Geometry check sheet. Reference: the model listing, model coordinates, mm. A direction names the side the tool comes from. Coordinates: 2 decimals unless noted, no trailing zeros. Write each loop counter-clockwise with the first axis right and the second up, starting at its lowest first coordinate (ties: lowest second). Pieces come first, ordered by that corner, then holes. Notation, with made-up numbers: (12.5, 42.25) -> (69.5, 42.25) arc R26 cw to (69.5, 70.25) -> close; hole circle Ø9 at (-11, 70). An arc over 180 degrees is marked (long way). Answer in a Markdown table with one row per item. Add a question column.
Q1. Gauge pin test, flat end, axial feed: P1, Ø2, axis at x = 0, y = -22.225, coming from the -Z side. Record the tip position at first contact, or that the pin passes through.
Q2. Section check C-C, the plane z = 3. Count the separate pieces of the cut face and the enclosed holes in it, and give its area (3 significant figures).
Q3. Release check for a two-part mould opening along X. For faces 1 (the face through (-20.3, -20.11, 2.57)), 2 (the face through (12, -12, 5.207)), 3 (the face through (20.11, -20.3, 2.57)), 4 (the face through (16.71, 16.63, 2.57)) record: pulls with the +X half, pulls with the -X half, needs draft (parallel to the pull), parting line crosses it, or undercut.
Q4. Section check D-D, the plane y = 24.5. Record the boundary of the cut face in (x, z), and give its area (3 significant figures).
Q5. Tool access check on faces 5 (the face through (20.9, 7.283, 2.64)), 6 (the face through (12, -12, 0)). Record the directions out of +Z, -Z, +X, -X, +Y, -Y that give a thin tool (end or side, any length) a straight path to the whole face; none if there is none.
Q6. Thickness scan on line 1 (Y direction, x = 0, z = 3.1) (3 decimals); line 2 (Y direction, x = 21, z = 0.35); line 3 (Y direction, x = -7.5, z = 0.8). Record the ranges inside material, lowest first.
Q7. Section check A-A, the plane x = 0. Record the boundary of the cut face in (y, z) (3 decimals), and give its area (3 significant figures).
```python
from build123d import *

# Parameters (mm, degrees)
SKETCH4_R             = 28.575
BOSS_EXTRUDE2_DEPTH   = 5.207
SKETCH5_R             = 15.875
CUT_EXTRUDE5_DEPTH    = 6.207
CUT_EXTRUDE11_DEPTH   = 6.207
F_6_32_TAPPED_HOLE1_D = 2.7051


with BuildPart() as part:
    # Sketch4 → Boss-Extrude2 (new body)
    with BuildSketch(Plane.XY):
        Circle(SKETCH4_R)
    extrude(amount=BOSS_EXTRUDE2_DEPTH)

    # Sketch5 → Cut-Extrude5 (cut, through all)
    with BuildSketch(Plane.XY.offset(5.207)):
        Circle(SKETCH5_R)
    extrude(amount=-CUT_EXTRUDE5_DEPTH, mode=Mode.SUBTRACT)

    # Sketch8 → Cut-Extrude11 (cut, through all)
    with BuildSketch(Plane.XY.offset(5.207)):
        Polygon((32.367148217, 14.781549861), (13.593916116, 7.005422516), (14.565932035, 4.658768503), (33.339164135, 12.434895849), align=None)
        Polygon((12.351510066, 26.500513186), (10.004856053, 27.472529104), (9.518848094, 26.299202097), (11.865502107, 25.327186179), align=None)
        Polygon((-10.004856053, 27.472529104), (-12.351510066, 26.500513186), (-11.865502107, 25.327186179), (-9.518848094, 26.299202097), align=None)
        Polygon((-26.500513186, 12.351510066), (-27.472529104, 10.004856053), (-26.299202097, 9.518848094), (-25.327186179, 11.865502107), align=None)
        Polygon((-27.472529104, -10.004856053), (-26.500513186, -12.351510066), (-25.327186179, -11.865502107), (-26.299202097, -9.518848094), align=None)
        Polygon((-12.351510066, -26.500513186), (-10.004856053, -27.472529104), (-9.518848094, -26.299202097), (-11.865502107, -25.327186179), align=None)
        Polygon((10.004856053, -27.472529104), (12.351510066, -26.500513186), (11.865502107, -25.327186179), (9.518848094, -26.299202097), align=None)
        Polygon((26.500513186, -12.351510066), (27.472529104, -10.004856053), (26.299202097, -9.518848094), (25.327186179, -11.865502107), align=None)
    extrude(amount=-CUT_EXTRUDE11_DEPTH, mode=Mode.SUBTRACT)

    # #6-32 Tapped Hole1 (through all)
    with Locations(Plane.XY.offset(5.207)):
        with Locations((22.225, 0), (15.715448212, -15.715448212), (0, -22.225), (-15.715448212, -15.715448212), (-22.225, 0), (-15.715448212, 15.715448212), (0, 22.225), (15.715448212, 15.715448212)):
            Hole(F_6_32_TAPPED_HOLE1_D / 2)


solid = part.part
```
Calculated:
| question | item | result |
|---|---|---|
| 1 | P1 | passes through |
| 2 | separate pieces | 1 |
| 2 | enclosed holes | 8 |
| 2 | area | 1,680 mm² |
| 3 | face 1 | pulls with the -X half |
| 3 | face 2 | needs draft |
| 3 | face 3 | pulls with the +X half |
| 3 | face 4 | undercut |
| 4 | outline | (-14.71, 0) -> (14.71, 0) -> (14.71, 5.21) -> (-14.71, 5.21) -> close |
| 4 | area | 153 mm² |
| 5 | face 5 | +Z, -Z |
| 5 | face 6 | -Z, +X, -X, +Y, -Y |
| 6 | line 1 | y = -28.575 to -23.578, -20.872 to -15.875, 15.875 to 20.872, 23.578 to 28.575 |
| 6 | line 2 | y = -19.38 to -0.57, 0.57 to 7.32, 10.07 to 19.38 |
| 6 | line 3 | y = -27.57 to -13.99, 13.99 to 27.57 |
| 7 | outline | (-28.575, 0) -> (-23.578, 0) -> (-23.578, 5.207) -> (-28.575, 5.207) -> close; (-20.872, 0) -> (-15.875, 0) -> (-15.875, 5.207) -> (-20.872, 5.207) -> close; (15.875, 0) -> (20.872, 0) -> (20.872, 5.207) -> (15.875, 5.207) -> close; (23.578, 0) -> (28.575, 0) -> (28.575, 5.207) -> (23.578, 5.207) -> close |
| 7 | area | 104 mm² |
